For this review, take the finished solid that the model builds, in its own axes (mm). Give positions to 0.01 mm unless a question says otherwise; leave off trailing zeros. Loops run counter-clockwise (first coordinate to the right, second up) from the corner with the lowest first, then second, coordinate; pieces in that order, holes last.
```python
from build123d import *

# Parameters (mm, degrees)
SKETCH1_R               = 90
SKETCH1_R_2             = 80
BOSS_EXTRUDE1_DEPTH     = 40
CUT_EXTRUDE1_START      = -70
CUT_EXTRUDE1_DEPTH      = 70
SKETCH3_R               = 1.5
SKETCH3_R_2             = 1.75
CUT_EXTRUDE2_DEPTH      = 212
CHAMFER1_SIZE           = 2
CUT_EXTRUDE4_DEPTH      = 133.875882032
CUT_EXTRUDE4_DEPTH_BACK = 10
SKETCH4_W               = 1
SKETCH4_H               = 86.76850885


with BuildPart() as part:
    # Sketch1 → Boss-Extrude1 (new body)
    with BuildSketch(Plane(origin=(0, 0, 0), x_dir=(1, 0, 0), z_dir=(0, 1, 0))):
        with Locations(Location((0, 0, 0), (0, 0, 270))):
            Circle(SKETCH1_R)
        with Locations(Location((0, 0, 0), (0, 0, 270))):
            Circle(SKETCH1_R_2, mode=Mode.SUBTRACT)
    extrude(amount=BOSS_EXTRUDE1_DEPTH)

    # Sketch2 → Cut-Extrude1 (cut)
    with BuildSketch(Plane(origin=(0, 40, 0), x_dir=(1, 0, 0), z_dir=(0, 1, 0)).offset(CUT_EXTRUDE1_START)):
        with BuildLine():
            Line((-89.196412484, 12), (-89.196412484, -12))
            ThreePointArc((-89.196412484, -12), (-90, 0), (-89.196412484, 12))
        make_face()
        with BuildLine():
            Line((89.196412484, 12), (89.196412484, -12))
            ThreePointArc((89.196412484, -12), (90, 0), (89.196412484, 12))
        make_face()
    extrude(amount=CUT_EXTRUDE1_DEPTH, mode=Mode.SUBTRACT)

    # Sketch3 → Cut-Extrude2 (cut)
    with BuildSketch(Plane.ZY.offset(89.196412484)):
        with Locations((6.717514421, 26.717514421)):
            Circle(SKETCH3_R)
        with Locations((-5.656854249, 25.656854249)):
            Circle(SKETCH3_R)
        with Locations((-6.717514421, 13.282485579)):
            Circle(SKETCH3_R)
        with Locations((5.656854249, 14.343145751)):
            Circle(SKETCH3_R)
        with Locations((0, 20)):
            Circle(SKETCH3_R_2)
    extrude(amount=-CUT_EXTRUDE2_DEPTH, mode=Mode.SUBTRACT)

    # Chamfer1
    chamfer1_edges = [part.edges().sort_by_distance(p)[0] for p in [
        (89.196412484, 13.282485579, -8.217514421),
        (-89.196412484, 13.282485579, -8.217514421),
        (89.196412484, 26.717514421, 5.217514421),
        (-89.196412484, 26.717514421, 5.217514421),
        (89.196412484, 14.343145751, 4.156854249),
        (-89.196412484, 14.343145751, 4.156854249),
        (89.196412484, 25.656854249, -7.156854249),
        (-89.196412484, 25.656854249, -7.156854249),
    ]]
    chamfer(chamfer1_edges, length=CHAMFER1_SIZE)

    # Sketch4 → Cut-Extrude4 (cut, two sides: drawn at the far end of the back side and taken through both)
    with BuildSketch(Plane(origin=(0, 0, 0), x_dir=(1, 0, 0), z_dir=(0, 1, 0)).offset(-CUT_EXTRUDE4_DEPTH_BACK)):
        with Locations((0, 48.982222738)):
            Rectangle(SKETCH4_W, SKETCH4_H)
    extrude(amount=CUT_EXTRUDE4_DEPTH + CUT_EXTRUDE4_DEPTH_BACK, mode=Mode.SUBTRACT)


solid = part.part
```
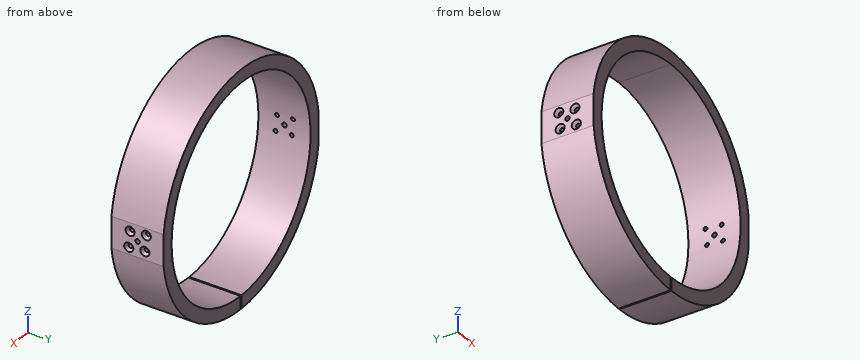
Q1. Consider section A-A on x = -27. Give the boundary of the cut face in (y, z), plus the area to 3 significant figures.
Answers:
outline: (0, -85.85) - (40, -85.85) - (40, -75.31) - (0, -75.31) - close; (0, 75.31) - (40, 75.31) - (40, 85.85) - (0, 85.85) - close
area: 844 mm2
Q2. For pin 1 Ø1 at (x, y) = (35.5, 10) entering from -Z; pin 2 Ø5 at (y, z) = (25.66, -5.66) entering from -X; pin 3 Ø2 at (x, y) = (-28, 19) entering from +Z, all flat-tipped, find the tip position at first contact; note any pin that passes through.
Answers:
pin 1: stops at z = -82.92
pin 2: stops at x = -88.2
pin 3: stops at z = 85.85
Q3. For probe 1 along Y at (x, z) = (-85.5, 0); probe 2 along Z at (x, y) = (-2, 29) (3 decimals); probe 3 along Z at (x, y) = (12, 6.5), list the stretches that pass through material, from the lowest coordinate up.
Answers:
probe 1: y = 0 to 18.25, 21.75 to 40
probe 2: z = -89.978 to -79.975, 79.975 to 89.978
probe 3: z = -89.2 to -79.09, 79.09 to 89.2
Q4. Consider section B-B on z = 19. Give the boundary of the cut face in (x, y).
Answers:
outline: (-87.97, 0) - (-77.71, 0) - (-77.71, 40) - (-87.97, 40) - close; (77.71, 0) - (87.97, 0) - (87.97, 40) - (77.71, 40) - close
Q5. Consider section C-C on y = 35.5. Give the boundary of the cut face in (x, z), plus the area to 3 significant figures.
Answers:
outline: (-89.2, -12) arc R90 ccw to (-0.5, -90) - (-0.5, -80) arc R80 cw (long way) to (0.5, -80) - (0.5, -90) arc R90 ccw to (89.2, -12) - (89.2, 12) arc R90 ccw to (-89.2, 12) - close
area: 5,300 mm2
